Design review of the part built by this model. Coordinates are the model's own, in mm. A direction names the side the tool comes from. Coordinates: 2 decimals unless noted, no trailing zeros. Loops run counter-clockwise (first coordinate to the right, second up) from the corner with the lowest first, then second, coordinate; pieces in that order, holes last.
Q1. For P1, Ø0.9, axis at y = 1.5, z = -26.5, coming from the +X side; P2, Ø0.9, axis at y = 2, z = -20.5, coming from the -X side, all flat-tipped, find the tip position at first contact; note any pin that passes through.
Q2. Add section D-D on z = -15.5. Give the boundary of the cut face in (x, y), and give its area (3 significant figures).
Q3. Add section B-B on x = -62.5. Give the boundary of the cut face in (y, z).
Q4. Wall thickness on probe 1 along X at (y, z) = (1.4, -27); probe 2 along X at (y, z) = (0.55, -5); probe 3 along Z at (x, y) = (59, 2.25): over which ranges is each line inside the solid? List them lowest first.
Q5. Add section C-C on y = 0.75. Give the number of separate pieces and of enclosed holes in the cut face, and give its area (3 significant figures).
Q6. Draft analysis for pull direction Z (two halves, no side actions). For faces 5 (the face through (49, 1, 36.935)), 6 (the face through (0, 1, -38.065)), 7 (the face through (66.69, 2, -1)), state which applies: released by +Z, released by -Z, zero draft, split by the parting line, or undercut.
Q7. Machinability: for faces 1 (the face through (74, 1, 11.935)), 2 (the face through (74, 1, -13.065)), 3 (the face through (-73, 1, -13.065)), 4 (the face through (1, 2, 33.935)), which of the approach directions +Z, -Z, +X, -X, +Y, -Y give a long, thin tool a straight path to every point of the face, cutting with its end or side? Answer none if there is none.
Q8. Add section A-A on z = 0.5. Give the boundary of the cut face in (x, y).
Autodesk Inventor part; units mm, degrees
ref_plane "YZ Plane" through (0, 0, 0) normal (1, 0, 0) x (0, 1, 0)
ref_plane "XZ Plane" through (0, 0, 0) normal (0, 1, 0) x (-1, 0, 0)
ref_plane "XY Plane" through (0, 0, 0) normal (0, 0, 1) x (1, 0, 0)
sketch "Sketch1" plane through (0, 0, 0) normal (0, 1, 0) x (-1, 0, 0)
  line L0 (71.1097, -38.0648) -> (71.1097, -13.0648)
  line L1 (71.1097, -13.0648) -> (74.1097, -13.0648)
  line L2 (74.1097, -13.0648) -> (74.1097, 11.9352)
  line L3 (74.1097, 11.9352) -> (71.1097, 11.9352)
  line L4 (71.1097, 11.9352) -> (71.1097, 36.9352)
  line L5 (-72.8903, -38.0648) -> (-72.8903, -13.0648)
  line L6 (-72.8903, 36.9352) -> (-72.8903, 11.9352)
  line L7 (-72.8903, -13.0648) -> (-75.8903, -13.0648)
  line L8 (-75.8903, -13.0648) -> (-75.8903, 11.9352)
  line L9 (-75.8903, 11.9352) -> (-72.8903, 11.9352)
  line L10 (71.1097, -38.0648) -> (-72.8903, -38.0648)
  line L11 (71.1097, 36.9352) -> (-72.8903, 36.9352)
  point P0 (0, 0)
extrude "Extrusion1" add sketch "Sketch1" along normal blind 3
sketch "Sketch2" plane through (0, 3, 0) normal (0, 1, 0) x (1, 0, 0)
  line L0 (-74.1097, 13.0648) -> (-74.1097, -11.9352)
  line L1 (75.8903, -11.9352) -> (75.8903, 13.0648)
  line L2 (-71.1097, -36.9352) -> (72.8903, -36.9352)
  line L3 (-24.1097, -36.9352) -> (25.8903, -36.9352)
  line L4 (25.8903, -36.9352) -> (25.8903, -33.9352)
  line L5 (25.8903, -33.9352) -> (-24.1097, -33.9352)
  line L6 (-24.1097, -33.9352) -> (-24.1097, -36.9352)
  line L7 (72.8903, 38.0648) -> (-71.1097, 38.0648)
  point P0 (0, 0)
  dimension "d13" = 50
  dimension "d14" = 3
extrude "Extrusion2" cut sketch "Sketch2" against normal blind 30
sketch "Sketch3" plane through (0, 3, 0) normal (0, 1, 0) x (1, 0, 0)
  line L0 (-71.1097, -36.9352) -> (-24.1097, -36.9352)
  line L1 (-74.1097, 13.0648) -> (-74.1097, -11.9352)
  line L2 (-54.9097, 25.4648) -> (-64.9114, 25.4648)
  line L3 (-64.9114, 25.4648) -> (-64.9114, -24.8352)
  line L4 (-64.9114, -24.8352) -> (-54.9097, -24.8352)
  line L5 (-54.9097, -24.8352) -> (-54.9097, 25.4648)
  line L6 (56.6903, 25.4648) -> (66.6903, 25.4648)
  line L7 (66.6903, 25.4648) -> (66.6903, -24.8352)
  line L8 (66.6903, -24.8352) -> (56.6903, -24.8352)
  line L9 (56.6903, -24.8352) -> (56.6903, 25.4648)
  circle A0 centre (-34.6697, 22.9248) radius 2
  circle A1 centre (-35.9397, -22.2952) radius 2
  circle A2 centre (40.2603, 22.9248) radius 2
  circle A3 centre (46.6103, -22.2952) radius 2
  line L10 (-49.9097, 28.4648) -> (51.6903, 28.4648)
  line L11 (51.6903, 28.4648) -> (51.6903, 33.4648)
  line L12 (51.6903, 33.4648) -> (-49.9097, 33.4648)
  line L13 (-49.9097, 33.4648) -> (-49.9097, 28.4648)
  point P0 (0, 0)
  dimension "d32" = 4
  dimension "d35" = 4
  dimension "d38" = 4
  dimension "d39" = 4
extrude "Extrusion3" cut sketch "Sketch3" against normal blind 10
sketch "Sketch4" plane through (-49.9097, 3, -33.4648) normal (0, 0, 1) x (1, 0, 0)
  line L0 (0, 0) -> (101.6, 0)
  line L1 (0, 0) -> (101.6, 0)
  line L2 (101.6, 0) -> (101.6, -3)
  line L3 (101.6, -3) -> (0, -3)
  line L4 (0, -3) -> (0, 0)
  point P0 (49.9097, -3)
extrude "Extrusion4" add sketch "Sketch4" along normal blind 5.2375
sketch "Sketch5" plane through (0, 3, 0) normal (0, 1, 0) x (1, 0, 0)
  circle A0 centre (-34.6697, 22.9248) radius 2
  circle A1 centre (-34.6697, 22.9248) radius 2
  circle A2 centre (40.2603, 22.9248) radius 2
  circle A3 centre (40.2603, 22.9248) radius 2
  circle A4 centre (46.6103, -22.2952) radius 2
  circle A5 centre (46.6103, -22.2952) radius 2
  circle A6 centre (-35.9397, -22.2952) radius 2
  circle A7 centre (-35.9397, -22.2952) radius 2
  point P0 (0, 0)
extrude "Extrusion5" add sketch "Sketch5" against normal blind 3
sketch "Sketch6" plane through (0, 3, 0) normal (0, 1, 0) x (1, 0, 0)
  point P0 (0, 0)
sketch "Sketch7" plane through (0, 3, 0) normal (0, 1, 0) x (1, 0, 0)
  line L0 (-54.9097, -24.8352) -> (-54.9097, 25.4648)
  line L1 (56.6903, 25.4648) -> (56.6903, -24.8352)
  line L2 (72.8903, 38.0648) -> (-71.1097, 38.0648)
  line L3 (25.8903, -36.9352) -> (72.8903, -36.9352)
  line L4 (-74.1097, 13.0648) -> (-74.1097, -11.9352)
  line L5 (75.8903, -11.9352) -> (75.8903, 13.0648)
  line L6 (-64.9114, 25.4648) -> (-64.9114, -24.8352)
  line L7 (-64.9114, 25.4648) -> (-54.9097, 25.4648)
  line L8 (-54.9097, 25.4648) -> (-54.9097, 27.2348)
  line L9 (-54.9097, 27.2348) -> (-64.9114, 27.2348)
  line L10 (-64.9114, 27.2348) -> (-64.9114, 25.4648)
  line L11 (-64.9114, -24.8352) -> (-54.9097, -24.8352)
  line L12 (-54.9097, -24.8352) -> (-54.9097, -26.1052)
  line L13 (-54.9097, -26.1052) -> (-64.9114, -26.1052)
  line L14 (-64.9114, -26.1052) -> (-64.9114, -24.8352)
  line L15 (56.6903, -24.8352) -> (66.6903, -24.8352)
  line L16 (56.6903, -24.8352) -> (66.6903, -24.8352)
  line L17 (66.6903, -24.8352) -> (66.6903, -26.1052)
  line L18 (66.6903, -26.1052) -> (56.6903, -26.1052)
  line L19 (56.6903, -26.1052) -> (56.6903, -24.8352)
  line L20 (66.6903, 25.4648) -> (56.6903, 25.4648)
  line L21 (56.6903, 25.4648) -> (66.6903, 25.4648)
  line L22 (66.6903, 25.4648) -> (66.6903, 27.2348)
  line L23 (66.6903, 27.2348) -> (56.6903, 27.2348)
  line L24 (56.6903, 27.2348) -> (56.6903, 25.4648)
  circle A0 centre (-35.9397, -23.5652) radius 2
  circle A1 centre (46.6103, -23.5652) radius 2
  circle A2 centre (-34.6697, 24.6948) radius 2
  circle A3 centre (40.2603, 24.6948) radius 2
  circle A4 centre (16.1303, -18.4852) radius 2
  circle A5 centre (16.1303, 9.4148) radius 2
  point P0 (0, 0)
  dimension "d61" = 4
  dimension "d63" = 4
  dimension "d69" = 4
  dimension "d71" = 4
  dimension "d74" = 4
  dimension "d76" = 4
extrude "Extrusion6" cut sketch "Sketch7" against normal blind 3 contours L12 L13 L14 L11 | L7 L10 L9 L8 | L15 L17 L18 L19 | L24 L23 L22 L20 | A0 | A1 | A2 | A3 | A4 | A5
sketch "Sketch8" plane through (0, 3, 0) normal (0, 1, 0) x (1, 0, 0)
  point P0 (0, 0)
sketch "Sketch9" plane through (0, 3, 0) normal (0, 1, 0) x (1, 0, 0)
  circle A0 centre (46.6103, -23.5652) radius 2
  circle A1 centre (-35.9397, -23.5652) radius 2
  circle A2 centre (40.2603, 24.6948) radius 2
  point P0 (0, 0)
sketch "Sketch10" plane through (0, 3, 0) normal (0, 1, 0) x (1, 0, 0)
  line L0 (56.6903, 27.2348) -> (66.6903, 27.2348)
  line L1 (56.6903, 27.2348) -> (51.6903, 27.2348)
  line L2 (51.6903, 27.2348) -> (51.6903, -26.1052)
  line L3 (51.6903, -26.1052) -> (56.6903, -26.1052)
  line L4 (56.6903, -26.1052) -> (56.6903, 27.2348)
  line L5 (-54.9097, -26.1052) -> (-54.9097, 27.2348)
  line L6 (-54.9097, 27.2348) -> (-49.9097, 27.2348)
  line L7 (-49.9097, 27.2348) -> (-49.9097, -26.1052)
  line L8 (-49.9097, -26.1052) -> (-54.9097, -26.1052)
  line L9 (-54.9097, -26.1052) -> (-54.9097, 27.2348)
  point P0 (0, 0)
  dimension "d79" = 5
  dimension "d80" = 5
extrude "Extrusion7" cut sketch "Sketch10" against normal blind 10
properties part number "Level2 (Arduino)"
Entries:
1. P1: stops at x = 72.89
1. P2: stops at x = -71.11
2. outline: (-71.11, 0) - (-64.91, 0) - (-64.91, 3) - (-71.11, 3) - close; (-49.91, 0) - (51.69, 0) - (51.69, 3) - (-49.91, 3) - close; (66.69, 0) - (72.89, 0) - (72.89, 3) - (66.69, 3) - close
2. area: 342 mm2
3. outline: (0, -38.06) - (3, -38.06) - (3, -27.23) - (0, -27.23) - close; (0, 26.11) - (3, 26.11) - (3, 36.94) - (0, 36.94) - close
4. probe 1: x = -71.11 to -64.91, -49.91 to 51.69, 66.69 to 72.89
4. probe 2: x = -74.11 to -64.91, -49.91 to 51.69, 66.69 to 75.89
4. probe 3: z = -38.06 to -27.23, 26.11 to 36.94
5. separate pieces: 1
5. enclosed holes: 8
5. area: 9,120 mm2
6. face 5: released by +Z
6. face 6: released by -Z
6. face 7: undercut
7. face 1: +Z, +X, +Y, -Y
7. face 2: -Z, +X, +Y, -Y
7. face 3: -Z, -X, +Y, -Y
7. face 4: +Z, +Y, -Y
8. outline: (-74.11, 0) - (-64.91, 0) - (-64.91, 3) - (-74.11, 3) - close; (-49.91, 0) - (51.69, 0) - (51.69, 3) - (-49.91, 3) - close; (66.69, 0) - (75.89, 0) - (75.89, 3) - (66.69, 3) - close
